Part print with two shaded views. Sizes in mm from the minimum x, y, z corner. Round coordinates to 2 decimals unless told otherwise and drop trailing zeros. Loops run counter-clockwise (first coordinate to the right, second up) from the corner with the lowest first, then second, coordinate; pieces in that order, holes last. Notation, with made-up numbers: (-12.75, 29.5) - (34.25, 29.5) arc R16 ccw to (34.25, 55.5) - close; hole circle Ø10 at (13, 55). An arc over 180 degrees is marked (long way). Use a Markdown table: item, result.
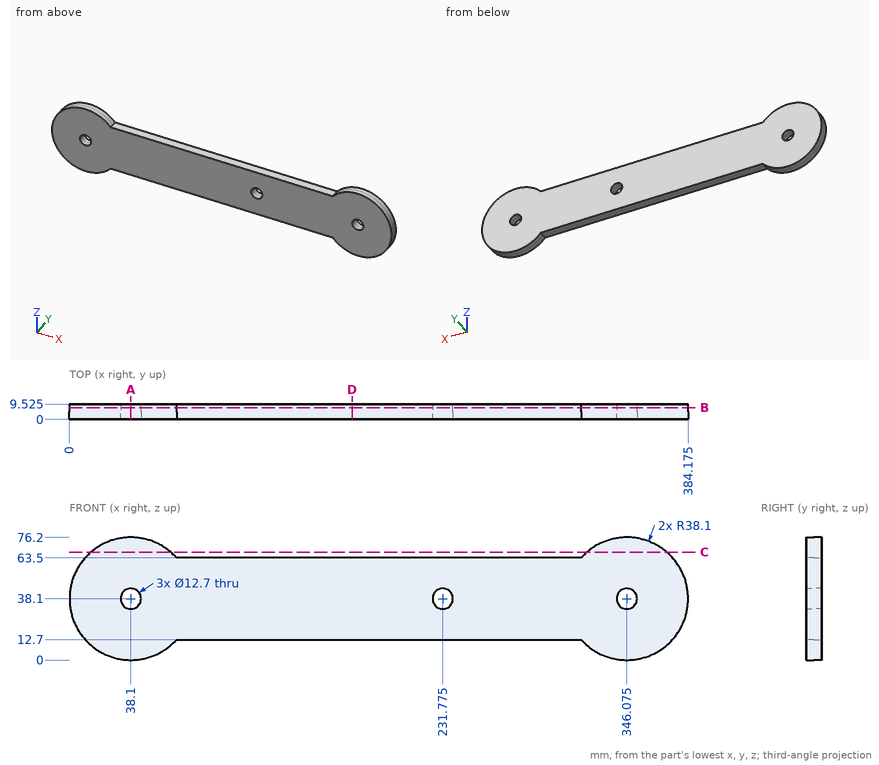
Q1. Cut at C-C, the plane z = 67. List the corners of the cut face in (x, y) (3 decimals), plus the area to 3 significant figures.
Results found:
| item | result |
|---|---|
| outline | (13.273, 0) - (62.927, 0) - (62.927, 9.525) - (13.273, 9.525) - close; (321.248, 0) - (370.902, 0) - (370.902, 9.525) - (321.248, 9.525) - close |
| area | 946 mm2 |
Q2. Cut at B-B, the plane y = 7.25. List the corners of the cut face in (x, z) (3 decimals).
Results found:
| item | result |
|---|---|
| outline | (66.498, 12.7) - (317.677, 12.7) arc R38.1 ccw (long way) to (317.677, 63.5) - (66.498, 63.5) arc R38.1 ccw (long way) to start; hole circle Ø12.7 at (38.1, 38.1); hole circle Ø12.7 at (231.775, 38.1); hole circle Ø12.7 at (346.075, 38.1) |
Q3. Cut at A-A, the plane x = 38.1. List the corners of the cut face in (y, z) (3 decimals).
Results found:
| item | result |
|---|---|
| outline | (0, 0) - (9.525, 0) - (9.525, 31.75) - (0, 31.75) - close; (0, 44.45) - (9.525, 44.45) - (9.525, 76.2) - (0, 76.2) - close |
Q4. Cut at D-D, the plane x = 175.5. List the corners of the cut face in (y, z) (3 decimals).
Results found:
| item | result |
|---|---|
| outline | (0, 12.7) - (9.525, 12.7) - (9.525, 63.5) - (0, 63.5) - close |
Q5. Probe line 1 (X direction, y = 6.75, z = 43); line 2 (X direction, y = 1, z = 34); line 3 (Z direction, x = 105, y = 6). List the from-to ranges inside material, lowest first.
Results found:
| item | result |
|---|---|
| line 1 | x = 0.32 to 34.06, 42.14 to 227.74, 235.81 to 342.04, 350.11 to 383.86 |
| line 2 | x = 0.22 to 33.25, 42.95 to 226.93, 236.62 to 341.23, 350.92 to 383.95 |
| line 3 | z = 12.7 to 63.5 |
Q6. Drop flat-ended pins along their axis: pin 1 (1.5 mm diameter, centred on x = 182, y = 4, fed in from -Z); pin 2 (1.5 mm diameter, centred on y = 3.5, z = 63.5, fed in from +X); pin 3 (16.5 mm diameter, centred on x = 346.075, z = 38.1, fed in from +Y) (3 decimals); pin 4 (3 mm diameter, centred on x = 154.5, y = 4.5, fed in from +Z). Give the stop position or say it passes through.
Results found:
| item | result |
|---|---|
| pin 1 | stops at z = 12.7 |
| pin 2 | stops at x = 375.13 |
| pin 3 | stops at y = 9.525 |
| pin 4 | stops at z = 63.5 |
